Design review of the part built by this model. Coordinates are the model's own, in mm. Round coordinates to 2 decimals unless told otherwise and drop trailing zeros.
Autodesk Inventor part; units mm, degrees
ref_plane "side_4d_XY" through (-20, 0, -330) normal (-1, 0, 0) x (0, 1, 0)
ref_plane "side_4d_YZ" through (-20, 0, -330) normal (0, 1, 0) x (0, 0, -1)
ref_plane "side_4d_ZX" through (-20, 0, -330) normal (0, 0, -1) x (-1, 0, 0)
sketch "Skizze_1" plane through (0, 0, 0) normal (0, 0, 1) x (1, 0, 0)
  arc A0 (-20, -17) -> (-17, -20) centre (-17, -17) ccw
  line L0 (-17, -20) -> (-4.1, -20)
  line L1 (-4.1, -20) -> (-4.1, -17)
  line L2 (-4.1, -17) -> (-10.5, -17)
  line L3 (-10.5, -17) -> (-10.5, -13.6627)
  arc A1 (-10.0314, -12.5314) -> (-10.5, -13.6627) centre (-8.9002, -13.6627) ccw
  line L4 (-10.0314, -12.5314) -> (-7.4645, -9.9645)
  arc A2 (-3.9289, -8.5) -> (-7.4645, -9.9645) centre (-3.9289, -13.5) ccw
  line L5 (-3.9289, -8.5) -> (3.9289, -8.5)
  arc A3 (7.4645, -9.9645) -> (3.9289, -8.5) centre (3.9289, -13.5) ccw
  line L6 (7.4645, -9.9645) -> (10.0314, -12.5314)
  arc A4 (10.5, -13.6627) -> (10.0314, -12.5314) centre (8.9002, -13.6627) ccw
  line L7 (10.5, -13.6627) -> (10.5, -17)
  line L8 (10.5, -17) -> (4.1, -17)
  line L9 (4.1, -17) -> (4.1, -20)
  line L10 (4.1, -20) -> (17, -20)
  arc A5 (17, -20) -> (20, -17) centre (17, -17) ccw
  line L11 (20, -17) -> (20, -4.1)
  line L12 (20, -4.1) -> (17, -4.1)
  line L13 (17, -4.1) -> (17, -10.5)
  line L14 (17, -10.5) -> (13.6627, -10.5)
  arc A6 (12.5314, -10.0314) -> (13.6627, -10.5) centre (13.6627, -8.9002) ccw
  line L15 (12.5314, -10.0314) -> (9.9645, -7.4645)
  arc A7 (8.5, -3.9289) -> (9.9645, -7.4645) centre (13.5, -3.9289) ccw
  line L16 (8.5, -3.9289) -> (8.5, 3.9289)
  arc A8 (9.9645, 7.4645) -> (8.5, 3.9289) centre (13.5, 3.9289) ccw
  line L17 (9.9645, 7.4645) -> (12.5314, 10.0314)
  arc A9 (13.6627, 10.5) -> (12.5314, 10.0314) centre (13.6627, 8.9002) ccw
  line L18 (13.6627, 10.5) -> (17, 10.5)
  line L19 (17, 10.5) -> (17, 4.1)
  line L20 (17, 4.1) -> (20, 4.1)
  line L21 (20, 4.1) -> (20, 17)
  arc A10 (20, 17) -> (17, 20) centre (17, 17) ccw
  line L22 (17, 20) -> (4.1, 20)
  line L23 (4.1, 20) -> (4.1, 17)
  line L24 (4.1, 17) -> (10.5, 17)
  line L25 (10.5, 17) -> (10.5, 13.6627)
  arc A11 (10.0314, 12.5314) -> (10.5, 13.6627) centre (8.9002, 13.6627) ccw
  line L26 (10.0314, 12.5314) -> (7.4645, 9.9645)
  arc A12 (3.9289, 8.5) -> (7.4645, 9.9645) centre (3.9289, 13.5) ccw
  line L27 (3.9289, 8.5) -> (-3.9289, 8.5)
  arc A13 (-7.4645, 9.9645) -> (-3.9289, 8.5) centre (-3.9289, 13.5) ccw
  line L28 (-7.4645, 9.9645) -> (-10.0314, 12.5314)
  arc A14 (-10.5, 13.6627) -> (-10.0314, 12.5314) centre (-8.9002, 13.6627) ccw
  line L29 (-10.5, 13.6627) -> (-10.5, 17)
  line L30 (-10.5, 17) -> (-4.1, 17)
  line L31 (-4.1, 17) -> (-4.1, 20)
  line L32 (-4.1, 20) -> (-17, 20)
  arc A15 (-17, 20) -> (-20, 17) centre (-17, 17) ccw
  line L33 (-20, 17) -> (-20, 4.1)
  line L34 (-20, 4.1) -> (-17, 4.1)
  line L35 (-17, 4.1) -> (-17, 10.5)
  line L36 (-17, 10.5) -> (-13.6627, 10.5)
  arc A16 (-12.5314, 10.0314) -> (-13.6627, 10.5) centre (-13.6627, 8.9002) ccw
  line L37 (-12.5314, 10.0314) -> (-9.9645, 7.4645)
  arc A17 (-8.5, 3.9289) -> (-9.9645, 7.4645) centre (-13.5, 3.9289) ccw
  line L38 (-8.5, 3.9289) -> (-8.5, -3.9289)
  arc A18 (-9.9645, -7.4645) -> (-8.5, -3.9289) centre (-13.5, -3.9289) ccw
  line L39 (-9.9645, -7.4645) -> (-12.5314, -10.0314)
  arc A19 (-13.6627, -10.5) -> (-12.5314, -10.0314) centre (-13.6627, -8.9002) ccw
  line L40 (-13.6627, -10.5) -> (-17, -10.5)
  line L41 (-17, -10.5) -> (-17, -4.1)
  line L42 (-17, -4.1) -> (-20, -4.1)
  line L43 (-20, -4.1) -> (-20, -17)
  circle A20 centre (0, 0) radius 6
extrude "Extrusion1" add sketch "Skizze_1" along normal blind 640
sketch "Sketch2" plane through (0, 0, 0) normal (0, 0, -1) x (1, 0, 0)
  point P0 (-15, -15)
hole "Drilling 1" at (-15, 15, 0) direction (0, 0, 1) diameter 5 depth 6000
sketch "Sketch3" plane through (0, 0, 0) normal (0, 0, -1) x (1, 0, 0)
  point P0 (15, -15)
hole "Drilling 2" at (15, 15, 0) direction (0, 0, 1) diameter 5 depth 6000
sketch "Sketch4" plane through (0, 0, 0) normal (0, 0, -1) x (1, 0, 0)
  point P0 (15, 15)
hole "Drilling 3" at (15, -15, 0) direction (0, 0, 1) diameter 5 depth 6000
sketch "Sketch5" plane through (0, 0, 0) normal (0, 0, -1) x (1, 0, 0)
  point P0 (-15, 15)
hole "Drilling 4" at (-15, -15, 0) direction (0, 0, 1) diameter 5 depth 6000
ref_plane "side_4d_XY" through (-20, 0, -330) normal (-1, 0, 0) x (0, 1, 0)
ref_plane "side_4d_YZ" through (-20, 0, -330) normal (0, 1, 0) x (0, 0, -1)
ref_plane "side_4d_ZX" through (-20, 0, -330) normal (0, 0, -1) x (-1, 0, 0)
ref_plane "side_1a_XY" through (0, 20, -330) normal (0, 1, 0) x (1, 0, 0)
ref_plane "side_1a_YZ" through (0, 20, -330) normal (1, 0, 0) x (0, 0, -1)
ref_plane "side_1a_ZX" through (0, 20, -330) normal (0, 0, -1) x (0, 1, 0)
ref_plane "side_2b_XY" through (20, 0, -330) normal (1, 0, 0) x (0, -1, 0)
ref_plane "side_2b_YZ" through (20, 0, -330) normal (0, -1, 0) x (0, 0, -1)
ref_plane "side_2b_ZX" through (20, 0, -330) normal (0, 0, -1) x (1, 0, 0)
ref_plane "side_3c_XY" through (0, -20, -330) normal (0, -1, 0) x (-1, 0, 0)
ref_plane "side_3c_YZ" through (0, -20, -330) normal (-1, 0, 0) x (0, 0, -1)
ref_plane "side_3c_ZX" through (0, -20, -330) normal (0, 0, -1) x (0, -1, 0)
ref_plane "end_XY" through (0, 0, -660) normal (0, 0, -1) x (1, 0, 0)
ref_plane "end_YZ" through (0, 0, -660) normal (1, 0, 0) x (0, -1, 0)
ref_plane "end_ZX" through (0, 0, -660) normal (0, -1, 0) x (0, 0, -1)
ref_plane "start_XY" through (0, 0, 0) normal (0, 0, 1) x (1, 0, 0)
ref_plane "start_YZ" through (0, 0, 0) normal (1, 0, 0) x (0, 1, 0)
ref_plane "start_ZX" through (0, 0, 0) normal (0, 1, 0) x (0, 0, 1)
properties part number "MayTec 1.11.040040.43S_Profile 40x40, 4E, S_660_Detail_(0;0,0,0)"
1) Add section A-A on z = 584.5. Count the separate pieces of the cut face and the enclosed holes in it, and give its area (3 significant figures).
2) For P1, Ø0.9, axis at y = 19, z = 299.5, coming from the -X side; P2, Ø4.5, axis at x = -15, y = -15, coming from the -Z side; P3, Ø1.5, axis at x = -18.5, z = 468, coming from the -Y side; P4, Ø4, axis at y = -1, z = 430, coming from the -X side, all flat-tipped, find the tip position at first contact; note any pin that passes through.
3) The part is to be moulded in two halves that separate along Y. For faces 1 (the face through (-11, -20, 316)), 2 (the face through (-6, 0, 316)), 3 (the face through (20, 10, 316)), say which applies: pulls with the +Y half, pulls with the -Y half, needs draft (parallel to the pull), parting line crosses it, or undercut.
4) For line 1 along Y through (x, z) = (15, 577.5); line 2 along Y through (x, z) = (-8, 68), list the stretches that pass through material, from the lowest coordinate up.
Computed:
1. separate pieces: 1
1. enclosed holes: 5
1. area: 674 mm2
2. P1: stops at x = -19.57
2. P2: passes through
2. P3: stops at y = -19.9
2. P4: stops at x = -8.5
3. face 1: pulls with the -Y half
3. face 2: undercut
3. face 3: needs draft
4. line 1: y = -20 to -17.5, -12.5 to -10.5, 10.5 to 12.5, 17.5 to 20
4. line 2: y = -20 to -17, -10.5 to 10.5, 17 to 20
